Verification items for the finished model (mm, model axes). A direction names the side the tool comes from. Give positions to 0.01 mm unless a question says otherwise; leave off trailing zeros. Loops run counter-clockwise (first coordinate to the right, second up) from the corner with the lowest first, then second, coordinate; pieces in that order, holes last. Notation, with made-up numbers: M 6.5,60 L 38.5,60 A27 ccw 38.5,91 Z; hole C 38.5,-23.75 d11. An arc over 180 degrees is marked long. Use CSV: the item, a comma, the result in double quotes.
from build123d import *

# Parameters (mm, degrees)
EXTRUDE_1_DEPTH     = 20
SKETCH_2_R          = 10
EXTRUDE_2_DEPTH     = 25
SKETCH_3_R          = 1
CUT_EXTRUDE_1_DEPTH = 4
SKETCH_4_R          = 3
EXTRUDE_3_DEPTH     = 2
SKETCH_5_R          = 1
EXTRUDE_4_DEPTH     = 0.5
EXTRUDE_6_DEPTH     = 3
SKETCH_7_R          = 3.5
EXTRUDE_7_DEPTH     = 3
EXTRUDE_8_DEPTH     = 7.6


with BuildPart() as part:
    # 草图1 → 凸台-拉伸1 (new body)
    with BuildSketch(Plane.XY):
        with BuildLine():
            Line((-6.31961233, 7.75), (6.31961233, 7.75))
            ThreePointArc((6.31961233, 7.75), (10, 0), (6.31961233, -7.75))
            Line((6.31961233, -7.75), (-6.31961233, -7.75))
            ThreePointArc((-6.31961233, -7.75), (-10, 0), (-6.31961233, 7.75))
        make_face()
    extrude(amount=EXTRUDE_1_DEPTH)

    # 草图2 → 凸台-拉伸2 (add)
    with BuildSketch(Plane.XY.offset(20)):
        with Locations(Location((0, 0, 0), (0, 0, 129.194967426))):
            Circle(SKETCH_2_R)
    extrude(amount=EXTRUDE_2_DEPTH)

    # 草图3 → 切除-拉伸1 (cut)
    with BuildSketch(Plane.XY.offset(45)):
        with Locations((0, 7.5)):
            Circle(SKETCH_3_R)
        with Locations((0, -7.5)):
            Circle(SKETCH_3_R)
    extrude(amount=-CUT_EXTRUDE_1_DEPTH, mode=Mode.SUBTRACT)

    # 草图4 → 凸台-拉伸3 (add)
    with BuildSketch(Plane(origin=(0, 0, 0), x_dir=(-1, 0, 0), z_dir=(0, 0, -1))):
        Circle(SKETCH_4_R)
    extrude(amount=EXTRUDE_3_DEPTH)

    # 草图5 → 凸台-拉伸4 (add)
    with BuildSketch(Plane(origin=(0, 0, 0), x_dir=(-1, 0, 0), z_dir=(0, 0, -1))):
        with Locations(Location((-7.6, -1, 0), (0, 0, 180))):
            Circle(SKETCH_5_R)
        with Locations(Location((7.6, 1, 0), (0, 0, 180))):
            Circle(SKETCH_5_R)
    extrude(amount=EXTRUDE_4_DEPTH)

    # 草图6 → 凸台-拉伸6 (add)
    with BuildSketch(Plane(origin=(0, 0, -0.5), x_dir=(-1, 0, 0), z_dir=(0, 0, -1))):
        with BuildLine():
            Line((-8.568245837, -1.25), (-6.631754163, -1.25))
            ThreePointArc((-6.631754163, -1.25), (-6.6, -1), (-6.631754163, -0.75))
            Line((-6.631754163, -0.75), (-8.568245837, -0.75))
            ThreePointArc((-8.568245837, -0.75), (-8.6, -1), (-8.568245837, -1.25))
        make_face()
        with BuildLine():
            Line((6.631754163, 0.75), (8.568245837, 0.75))
            ThreePointArc((8.568245837, 0.75), (8.6, 1), (8.568245837, 1.25))
            Line((8.568245837, 1.25), (6.631754163, 1.25))
            ThreePointArc((6.631754163, 1.25), (6.6, 1), (6.631754163, 0.75))
        make_face()
    extrude(amount=EXTRUDE_6_DEPTH)

    # 草图7 → 凸台-拉伸7 (add)
    with BuildSketch(Plane.XY.offset(45)):
        Circle(SKETCH_7_R)
    extrude(amount=EXTRUDE_7_DEPTH)

    # 草图9 → 凸台-拉伸8 (add)
    with BuildSketch(Plane.XY.offset(48)):
        with BuildLine():
            Line((-1.322875656, 1.5), (1.322875656, 1.5))
            ThreePointArc((1.322875656, 1.5), (0, -2), (-1.322875656, 1.5))
        make_face()
    extrude(amount=EXTRUDE_8_DEPTH)


solid = part.part
(1) Tool access check on faces 5 (the flat face through (0, 1.5, 52)), 6 (the cylindrical face through (-0.13, 8.49, 43.03)), 7 (the flat face through (0, 4, 0)). Record the directions out of +Z, -Z, +X, -X, +Y, -Y that give a thin tool (end or side, any length) a straight path to the whole face; none if there is none.
Calculated:
face 5,"+Z, +X, -X, +Y"
face 6,"+Z"
face 7,"-Z"
(2) Section check C-C on y = 5. Record the cut outline in (x, z), plus the area to 3 significant figures.
Calculated:
outline,"M -8.66,0 L 8.66,0 L 8.66,45 L -8.66,45 Z"
area,"779 mm²"
(3) Section check A-A on x = 0. Record the cut outline in (y, z), plus the area to 3 significant figures.
Calculated:
outline,"M -10,20 L -7.75,20 L -7.75,0 L -3,0 L -3,-2 L 3,-2 L 3,0 L 7.75,0 L 7.75,20 L 10,20 L 10,45 L 8.5,45 L 8.5,41 L 6.5,41 L 6.5,45 L 3.5,45 L 3.5,48 L 1.5,48 L 1.5,55.6 L -2,55.6 L -2,48 L -3.5,48 L -3.5,45 L -6.5,45 L -6.5,41 L -8.5,41 L -8.5,45 L -10,45 Z"
area,"854 mm²"
(4) Section check B-B on z = 40. Record the cut outline in (x, y), plus the area to 3 significant figures.
Calculated:
outline,"C 0,0 d20"
area,"314 mm²"
(5) Scan lines: L1, parallel to Y at x = 0, z = 42; L2, parallel to Z at x = 3, y = -4.5; L3, parallel to Y at x = -0.5, z = 2. Record each from-to range of solid material in increasing order. Write a range as from..to.
Calculated:
L1,"y = -10..-8.5, -6.5..6.5, 8.5..10"
L2,"z = 0..45"
L3,"y = -7.75..7.75"
(6) Depth check by flat-ended pin: pin 1 Ø5 at (x, y) = (5.5, 3.5) entering from -Z; pin 2 Ø4 at (x, z) = (3, 11) entering from +Y; pin 3 Ø1.3 at (x, z) = (0.5, 52.5) entering from +Y. Enter the tip coordinate at first touch or a pass-through.
Calculated:
pin 1,"stops at z = 0"
pin 2,"stops at y = 7.75"
pin 3,"stops at y = 1.5"
(7) Mould release check, pull along Y, two halves, no side actions. Record for faces 1 (the cylindrical face through (3.233, -1.341, 46.479)), 2 (the flat face through (3, 3, 45)), 3 (the flat face through (0, 8, 41)), 4 (the flat face through (0, -7, 41)): released by +Y, released by -Y, zero draft, split by the parting line, or undercut.
Calculated:
face 1,"split by the parting line"
face 2,"zero draft"
face 3,"undercut"
face 4,"undercut"
(8) Section check D-D on z = 52.5. Record the cut outline in (x, y), plus the area to 3 significant figures.
Calculated:
outline,"M -1.32,1.5 A2 ccw long 1.32,1.5 Z"
area,"11.7 mm²"
